Work out the finished part from the listing and answer in its coordinate system (mm). Face numbers are marked on the shaded views. A direction names the side the tool comes from. Round coordinates to 2 decimals unless told otherwise and drop trailing zeros. Write each loop counter-clockwise with the first axis right and the second up, starting at its lowest first coordinate (ties: lowest second). Pieces come first, ordered by that corner, then holes. Notation, with made-up numbers: M -40,10 L 10,10 A22 ccw 10,22 Z; hole C 9.25,25.5 d7. An arc over 180 degrees is marked long. Answer in a Markdown table with one row per item.
```python
from build123d import *

# Parameters (mm, degrees)
F0_R     = 2
F1_DEPTH = 4
F2_R     = 3.5
F3_DEPTH = 3
F5_DEPTH = 16
F6_W     = 6
F6_H     = 13
F6_W_2   = 17
F6_R     = 1
F7_DEPTH = 25
F8_R     = 5


with BuildPart() as f1:
    # F0 (on Top) → F1 (new body)
    with BuildSketch(Plane.XY):
        Polygon((0, 6.640602), (-25.017791, 6.640602), (-25.017791, -11.776076), (-19.303476, -75.663209), (0, -75.663209), (19.303476, -75.663209), (25.017791, -11.776076), (25.017791, 6.640602), align=None)
        with Locations((-15.75, 0)):
            Circle(F0_R, mode=Mode.SUBTRACT)
        with Locations((15.75, 0)):
            Circle(F0_R, mode=Mode.SUBTRACT)
    extrude(amount=F1_DEPTH)

    # F2 (on face) → F3 (cut)
    with BuildSketch(Plane.XY.offset(4)):
        with Locations((-15.75, 0)):
            Circle(F2_R)
        with Locations((15.75, 0)):
            Circle(F2_R)
    extrude(amount=-F3_DEPTH, mode=Mode.SUBTRACT)

    # F4 (on face) → F5 (join)
    with BuildSketch(Plane(origin=(0, 0, 0), x_dir=(1, 0, 0), z_dir=(0, 0, -1))):
        Polygon((19.303476, 75.663209), (-19.303476, 75.663209), (-19.661252, 71.663209), (19.661252, 71.663209), align=None)
    extrude(amount=F5_DEPTH)

    # F6 (on face) → F7 (cut)
    with BuildSketch(Plane.XZ.offset(75.663209)):
        with Locations((6.303476, -6.5)):
            Rectangle(F6_W, F6_H)
        with Locations((-5.196524, -6.5)):
            Rectangle(F6_W_2, F6_H)
        with Locations((-16.696524, -6.5)):
            Circle(F6_R)
        with Locations((12.303476, -6.5)):
            Circle(F6_R)
    extrude(amount=-F7_DEPTH, mode=Mode.SUBTRACT)

    # F8
    f8_edges = [f1.edges().sort_by_distance(p)[0] for p in [
        (25.017791, 6.640602, 2),
        (-25.017791, 6.640602, 2),
    ]]
    fillet(f8_edges, radius=F8_R)


solid = f1.part
```
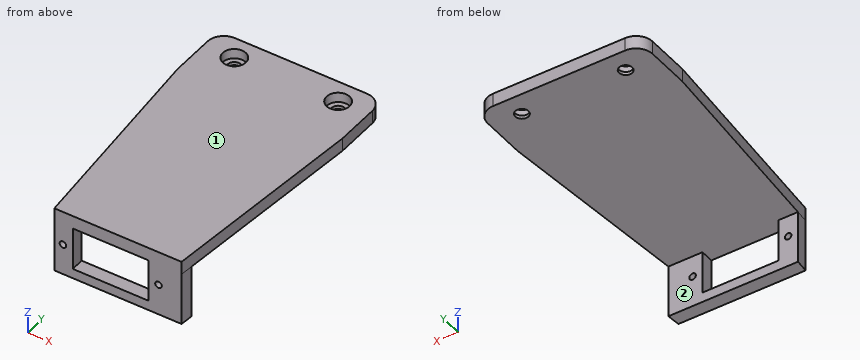
1. The part is cut by section D-D (x = 15.75). Determine the outline of the cut face in (y, z), plus the area to 3 significant figures.
Calculated:
| item | result |
|---|---|
| outline | M -75.66,-16 L -71.66,-16 L -71.66,0 L -2,0 L -2,1 L -3.5,1 L -3.5,4 L -75.66,4 Z; M 2,0 L 6.64,0 L 6.64,4 L 3.5,4 L 3.5,1 L 2,1 Z |
| area | 368 mm² |
2. The part is cut by section C-C (y = 0). Determine the outline of the cut face in (x, z).
Calculated:
| item | result |
|---|---|
| outline | M -25.02,0 L -17.75,0 L -17.75,1 L -19.25,1 L -19.25,4 L -25.02,4 Z; M -13.75,0 L 13.75,0 L 13.75,1 L 12.25,1 L 12.25,4 L -12.25,4 L -12.25,1 L -13.75,1 Z; M 17.75,0 L 25.02,0 L 25.02,4 L 19.25,4 L 19.25,1 L 17.75,1 Z |
3. The part is cut by section A-A (z = -3.75). Determine the outline of the cut face in (x, y).
Calculated:
| item | result |
|---|---|
| outline | M -19.66,-71.66 L -19.3,-75.66 L -13.7,-75.66 L -13.7,-71.66 Z; M 9.3,-75.66 L 19.3,-75.66 L 19.66,-71.66 L 9.3,-71.66 Z |
4. The part is cut by section B-B (x = -7). Determine the outline of the cut face in (y, z).
Calculated:
| item | result |
|---|---|
| outline | M -75.66,-16 L -71.66,-16 L -71.66,-13 L -75.66,-13 Z; M -75.66,0 L 6.64,0 L 6.64,4 L -75.66,4 Z |
5. Consider line 1 along X through (y, z) = (0, 0.6); line 2 along Y through (x, z) = (15.75, 2.5); line 3 along Z through (x, y) = (18, -59.5). Determine where each line is inside the solid, lowest interval first. Write a range as from..to.
Calculated:
| item | result |
|---|---|
| line 1 | x = -25.02..-17.75, -13.75..13.75, 17.75..25.02 |
| line 2 | y = -75.66..-3.5, 3.5..6.64 |
| line 3 | z = 0..4 |
6. Given pin 1 (5 mm diameter, centred on x = 10, z = -7.5, fed in from +Y); pin 2 (7.5 mm diameter, centred on x = 16.5, y = 0.5, fed in from +Z); pin 3 (25 mm diameter, centred on x = 4.5, y = -33.5, fed in from -Z); pin 4 (4.5 mm diameter, centred on y = -73.5, z = -4.5, fed in from +X), each flat-ended and moving along its own axis, determine where each tip first touches the part or whether it passes through.
Calculated:
| item | result |
|---|---|
| pin 1 | stops at y = -71.66 |
| pin 2 | stops at z = 4 |
| pin 3 | stops at z = 0 |
| pin 4 | stops at x = 19.66 |
7. A tool of negligible diameter and unlimited length cuts with its end or side. For the marked faces 1 and 2, from which of +Z, -Z, +X, -X, +Y, -Y can it reach the whole face along a straight path? Write none if from no direction.
Calculated:
| item | result |
|---|---|
| face 1 | +Z, +X, -X, +Y, -Y |
| face 2 | -Z, +X, -X, +Y |
